from build123d import *

# Parameters (mm, degrees)
ESQUISSE1_R                     = 17
BOSS_EXTRU_1_DEPTH              = 1.25
ENL_V_MAT_EXTRU_1_DEPTH         = 25.171263931
D_GAGEMENT_M2_51_D              = 2.7
R_P_TITION_CIRCULAIRE1_COUNT    = 3
DIAM_TRE_DU_PER_AGE_6_2_6_2_1_D = 6.2
BOSS_EXTRU_2_REACH              = 33.74
BOSS_EXTRU_2_END_RADIUS         = 17
BOSS_EXTRU_3_REACH              = 33.834
BOSS_EXTRU_3_END_RADIUS         = 17
R_P_TITION_CIRCULAIRE2_COUNT    = 3


with BuildPart() as part:
    # Esquisse1 → Boss.-Extru.1 (new, symmetric)
    with BuildSketch(Plane.XY):
        Circle(ESQUISSE1_R)
    extrude(amount=BOSS_EXTRU_1_DEPTH, both=True)

    # Esquisse2 → Enlèv. mat.-Extru.1 (cut, through all)
    with BuildSketch(Plane.XY.offset(1.25)):
        with BuildLine():
            Line((-9.85, 13.855594538), (-9.85, 8.227474827))
            ThreePointArc((-9.85, 8.227474827), (-9.475334198, 6.911057512), (-8.463636364, 5.989213437))
            ThreePointArc((-8.463636364, 5.989213437), (0, 4), (8.463636364, 5.989213437))
            ThreePointArc((8.463636364, 5.989213437), (9.475334198, 6.911057512), (9.85, 8.227474827))
            Line((9.85, 8.227474827), (9.85, 13.855594538))
            ThreePointArc((9.85, 13.855594538), (0, 17), (-9.85, 13.855594538))
        make_face()
    enl_v_mat_extru_1 = extrude(amount=-ENL_V_MAT_EXTRU_1_DEPTH, mode=Mode.SUBTRACT)

    # Dégagement M2.51 (through all)
    with Locations(Plane.XY.offset(1.25)):
        with Locations((12.384163274, 7.15)):
            d_gagement_m2_51 = Hole(D_GAGEMENT_M2_51_D / 2)

    # Répétition circulaire1: Enlèv. mat.-Extru.1, Dégagement M2.51 ×3 about axis
    r_p_tition_circulaire1_axis = Axis((0, 0, 0), (0, 0, 1))
    add([enl_v_mat_extru_1.rotate(r_p_tition_circulaire1_axis, i * 360 / R_P_TITION_CIRCULAIRE1_COUNT) for i in range(1, R_P_TITION_CIRCULAIRE1_COUNT)], mode=Mode.SUBTRACT)
    add([d_gagement_m2_51.rotate(r_p_tition_circulaire1_axis, i * 360 / R_P_TITION_CIRCULAIRE1_COUNT) for i in range(1, R_P_TITION_CIRCULAIRE1_COUNT)], mode=Mode.SUBTRACT)

    # Diamètre du perçage Ø6.2 (6.2)1 (through all)
    with Locations(Plane.XY.offset(1.25)):
        with Locations((0, 0)):
            Hole(DIAM_TRE_DU_PER_AGE_6_2_6_2_1_D / 2)

    # Boss.-Extru.2: up to this cylinder (the profile starts inside it)
    boss_extru_2_end = Plane(origin=(0, 0, 1.885519), z_dir=(0, 0, -1)) * Cylinder(BOSS_EXTRU_2_END_RADIUS, 102.48, mode=Mode.PRIVATE)
    # Esquisse8 → Boss.-Extru.2 (add, up to the surface)
    with BuildSketch(Plane(origin=(-9.85, 0, 0), x_dir=(0, 0, -1), z_dir=(1, 0, 0)), mode=Mode.PRIVATE) as boss_extru_2_sk1:
        Polygon((-1.25, 11.467766953), (-2.75, 12.967766953), (-2.75, 13.855594538), (-1.25, 13.855594538), align=None)
    boss_extru_2_tool1 = extrude(boss_extru_2_sk1.sketch, amount=-BOSS_EXTRU_2_REACH, mode=Mode.PRIVATE) & boss_extru_2_end
    boss_extru_2 = boss_extru_2_tool1.solids().sort_by_distance((-9.85, 12.97944, 1.885519))[0]
    add(boss_extru_2)

    # Boss.-Extru.3: up to this cylinder (the profile starts inside it)
    boss_extru_3_end = Plane(origin=(0, 0, 1.905844), z_dir=(0, 0, -1)) * Cylinder(BOSS_EXTRU_3_END_RADIUS, 102.668, mode=Mode.PRIVATE)
    # Esquisse9 → Boss.-Extru.3 (add, up to the surface)
    with BuildSketch(Plane.ZY.offset(-9.85), mode=Mode.PRIVATE) as boss_extru_3_sk1:
        Polygon((1.25, 13.855594538), (2.75, 13.855594538), (2.75, 12.614213562), (1.25, 11.114213562), align=None)
    boss_extru_3_tool1 = extrude(boss_extru_3_sk1.sketch, amount=-BOSS_EXTRU_3_REACH, mode=Mode.PRIVATE) & boss_extru_3_end
    boss_extru_3 = boss_extru_3_tool1.solids().sort_by_distance((9.85, 12.812826, 1.905844))[0]
    add(boss_extru_3)

    # Répétition circulaire2: Boss.-Extru.2, Boss.-Extru.3 ×3 about axis
    r_p_tition_circulaire2_axis = Axis((0, 0, 0), (0, 0, 1))
    add([boss_extru_2.rotate(r_p_tition_circulaire2_axis, i * 360 / R_P_TITION_CIRCULAIRE2_COUNT) for i in range(1, R_P_TITION_CIRCULAIRE2_COUNT)])
    add([boss_extru_3.rotate(r_p_tition_circulaire2_axis, i * 360 / R_P_TITION_CIRCULAIRE2_COUNT) for i in range(1, R_P_TITION_CIRCULAIRE2_COUNT)])


solid = part.part
Source: CAD feature listing. Evaluate the final solid. Frame: model axes, mm. A direction names the side the tool comes from. Coordinates: 2 decimals unless noted, no trailing zeros. Loops run counter-clockwise (first coordinate to the right, second up) from the corner with the lowest first, then second, coordinate; pieces in that order, holes last. Notation, with made-up numbers: M -36.75,82 L -30.75,82 A16 ccw -30.75,94 Z; hole C -17.5,54.25 d7. An arc over 180 degrees is marked long. Answer in a Markdown table with one row per item.
Q1. Section A-A on x = 0. Return the cut outline in (y, z), plus the area to 4 significant figures.
Answers below:
| item | result |
|---|---|
| outline | M -17,-1.25 L -15.65,-1.25 L -15.65,1.25 L -17,1.25 Z; M -12.95,-1.25 L -3.1,-1.25 L -3.1,1.25 L -12.95,1.25 Z; M 3.1,-1.25 L 4,-1.25 L 4,1.25 L 3.1,1.25 Z |
| area | 30.25 mm^2 |
Q2. First-contact query: pin 1 (2 mm diameter, centred on y = 10, z = 0.5, fed in from +X); pin 2 (2 mm diameter, centred on x = 6, y = 1, fed in from +Z). Flat tips, straight axial feed; report the tip coordinate or a pass-through.
Answers below:
| item | result |
|---|---|
| pin 1 | stops at x = 14.42 |
| pin 2 | stops at z = 1.25 |
Q3. Section D-D on z = 1.8. Return the cut outline in (x, y), plus the area to 3 significant figures.
Answers below:
| item | result |
|---|---|
| outline | M -16.92,1.6 L -15.03,2.7 L -16.29,4.88 A17 ccw Z; M -12.02,12.02 L -9.85,12.02 L -9.85,13.86 A17 ccw Z; M -7.07,-15.46 A17 ccw -4.4,-16.42 L -5.48,-14.54 Z; M 3.92,-16.54 A17 ccw 7.07,-15.46 L 5.18,-14.36 Z; M 9.85,11.66 L 12.37,11.66 A17 ccw 9.85,13.86 Z; M 15.33,2.52 L 16.92,1.6 A17 ccw 16.42,4.4 Z |
| area | 15.2 mm^2 |
Q4. Section C-C on y = 0. Return the cut outline in (x, z), plus the area to 3 significant figures.
Answers below:
| item | result |
|---|---|
| outline | M -4.79,-1.25 L -3.1,-1.25 L -3.1,1.25 L -4.79,1.25 Z; M 3.1,-1.25 L 4.79,-1.25 L 4.79,1.25 L 3.1,1.25 Z |
| area | 8.47 mm^2 |
Q5. Set-up query: faces 4 (the flat face through (14.5, 3, 0.3)), 5 (the flat face through (4.6, -14.03, 0.33)), 6 (the cylindrical face through (3.53, -1.89, 0.02)), 7 (the cylindrical face through (-1.257, -11.678, 0.018)). Return all of +Z, -Z, +X, -X, +Y, -Y with unobstructed straight access to the full face (end or side cutting, diameter ignored); none if empty.
Answers below:
| item | result |
|---|---|
| face 4 | +Z, -Z, -Y |
| face 5 | +Z, -Z, +X |
| face 6 | +Z, -Z |
| face 7 | +Z, -Z, -X |
Q6. Ray query, probe 1 along Y at (x, z) = (0, 0.4); probe 2 along X at (y, z) = (11, -0.65); probe 3 along X at (y, z) = (2, 0.3). Return the intervals inside material, ascending. Write a range as from..to.
Answers below:
| item | result |
|---|---|
| probe 1 | y = -17..-15.65, -12.95..-3.1, 3.1..4 |
| probe 2 | x = -12.96..-9.85, 9.85..12.96 |
| probe 3 | x = -16.88..-16.24, -6.55..-2.37, 2.37..6.55, 16.24..16.88 |
Q7. Section B-B on x = 6.5. Return the cut outline in (y, z), plus the area to 3 significant figures.
Answers below:
| item | result |
|---|---|
| outline | M -15.71,-1.25 L -15.13,-1.25 L -15.13,2.75 L -15.71,2.75 Z; M 1.95,-1.25 L 5.15,-1.25 L 5.15,1.25 L 1.95,1.25 Z |
| area | 10.3 mm^2 |
Q8. Draft query along X for faces 1 (the flat face through (-2, 3, 1.25)), 2 (the flat face through (-10.88, 12.04, 1.82)), 3 (the cylindrical face through (1.238, -11.644, 0.018)). Return one class per face: pulls with the +X half, pulls with the -X half, needs draft (parallel to the pull), parting line crosses it, or undercut.
Answers below:
| item | result |
|---|---|
| face 1 | undercut |
| face 2 | needs draft |
| face 3 | pulls with the +X half |
